Verification items for the finished model (mm, model axes). A direction names the side the tool comes from. Coordinates: 2 decimals unless noted, no trailing zeros. Order: outer loops, then holes, each group sorted by start corner. A loop starts at its lowest first (then second) coordinate and runs counter-clockwise, first axis right, second up. Notation, with made-up numbers: (66.5, 74) -> (80.5, 74) arc R22 ccw to (80.5, 85) -> close; hole circle Ø5 at (-21, -33). An arc over 180 degrees is marked (long way). Use CSV: the item, a comma, the result in double quotes. Start each with the question number.
1) Tool access check on faces 4 (the flat face through (-2, -36, 7)), 5 (the flat face through (-1, 3, -6)), 6 (the flat face through (49, -36, -8)), 7 (the cylindrical face through (44.536, 1.521, -6.325)). Record the directions out of +Z, -Z, +X, -X, +Y, -Y that give a thin tool (end or side, any length) a straight path to the whole face; none if there is none.
2) Scan lines: line 1 along X through (y, z) = (1.15, -6); line 2 along Y through (x, z) = (47.8, -5); line 3 along Y through (x, z) = (-37.5, -2.5). Record each from-to range of solid material in increasing order.
3) Sectioned sample at D-D on y = -37. Record the boundary of the cut face in (x, z), then the cut area to 3 significant figures.
4) Release check for a two-part mould opening along Y. For faces 1 (the cylindrical face through (-41.11, -60.03, 8.52)), 2 (the cylindrical face through (0.7, 2.39, 6.58)), 3 (the flat face through (-1, -38, 10)) record: released by +Y, released by -Y, zero draft, split by the parting line, or undercut.
5) Sectioned sample at C-C on z = 0.75. Record the boundary of the cut face in (x, y).
6) Sectioned sample at B-B on y = -55.27. Record the boundary of the cut face in (x, z), then the cut area to 3 significant figures.
7) Go/stop test with flat-tipped pins: pin 1 (2.5 mm diameter, centred on x = -23.5, y = -2, fed in from -Z); pin 2 (1.5 mm diameter, centred on x = 19, z = 5.5, fed in from -Y); pin 3 (1 mm diameter, centred on x = 38.5, z = -4, fed in from -Y); pin 4 (1.8 mm diameter, centred on x = -40, y = -61.04, fed in from +Z). Record where each tip stops, or that it passes through.
from build123d import *

# Parameters (mm, degrees)
SKETCH1_W           = 100
SKETCH1_H           = 20
BOSS_EXTRUDE1_DEPTH = 3
CUT_EXTRUDE1_REACH  = 53.078
SKETCH2_R           = 1.5
LPATTERN1_COUNT     = 2
LPATTERN1_PITCH     = 92
SKETCH3_W           = 100
SKETCH3_H           = 3
BOSS_EXTRUDE2_DEPTH = 68.54
SKETCH4_W           = 100
SKETCH4_H           = 5
BOSS_EXTRUDE3_DEPTH = 5
SKETCH5_W           = 100
SKETCH5_H           = 12
BOSS_EXTRUDE4_DEPTH = 3
FILLET4_R           = 12
SKETCH6_W           = 3
SKETCH6_H           = 63.54
BOSS_EXTRUDE5_DEPTH = 15
CUT_EXTRUDE2_REACH  = 123.646
SKETCH7_R           = 1.5
CUT_EXTRUDE3_REACH  = 89.165
SKETCH8_R           = 1.5
LPATTERN2_COUNT     = 2
LPATTERN2_PITCH     = 80


with BuildPart() as part:
    # Sketch1 → Boss-Extrude1 (new body)
    with BuildSketch(Plane(origin=(0, 0, 0), x_dir=(1, 0, 0), z_dir=(0, 1, 0))):
        Rectangle(SKETCH1_W, SKETCH1_H)
    extrude(amount=BOSS_EXTRUDE1_DEPTH)

    # Sketch2 → Cut-Extrude1 (cut, up to next)
    with BuildSketch(Plane(origin=(0, 3, 0), x_dir=(1, 0, 0), z_dir=(0, 1, 0)), mode=Mode.PRIVATE) as cut_extrude1_sk1:
        with Locations(Location((-46, 6, 0), (0, 0, 270))):
            Circle(SKETCH2_R)
    cut_extrude1_tool1 = extrude(cut_extrude1_sk1.sketch, amount=-CUT_EXTRUDE1_REACH, mode=Mode.PRIVATE) & part.part
    cut_extrude1 = cut_extrude1_tool1.solids().sort_by_distance((-46, 3, -6))[0]
    add(cut_extrude1, mode=Mode.SUBTRACT)

    # LPattern1: Cut-Extrude1 ×2
    with Locations(*[(i * LPATTERN1_PITCH, 0, 0) for i in range(1, LPATTERN1_COUNT)]):
        add(cut_extrude1, mode=Mode.SUBTRACT)

    # Sketch3 → Boss-Extrude2 (add)
    with BuildSketch(Plane.XZ):
        with Locations((0, 8.5)):
            Rectangle(SKETCH3_W, SKETCH3_H)
    extrude(amount=BOSS_EXTRUDE2_DEPTH)

    # Sketch4 → Boss-Extrude3 (add)
    with BuildSketch(Plane(origin=(0, 0, 7), x_dir=(-1, 0, 0), z_dir=(0, 0, -1))):
        with Locations((0, -2.5)):
            Rectangle(SKETCH4_W, SKETCH4_H)
    extrude(amount=BOSS_EXTRUDE3_DEPTH)

    # Sketch5 → Boss-Extrude4 (add)
    with BuildSketch(Plane(origin=(0, 3, 0), x_dir=(1, 0, 0), z_dir=(0, 1, 0))):
        with Locations((0, -4)):
            Rectangle(SKETCH5_W, SKETCH5_H)
    extrude(amount=BOSS_EXTRUDE4_DEPTH)

    # Fillet4
    fillet4_edges = [part.edges().sort_by_distance(p)[0] for p in [
        (0, 6, 10),
    ]]
    fillet(fillet4_edges, radius=FILLET4_R - 0.0001)  # a hair under: the kernel refuses the full size

    # Sketch6 → Boss-Extrude5 (add)
    with BuildSketch(Plane(origin=(0, 0, 7), x_dir=(-1, 0, 0), z_dir=(0, 0, -1))):
        with Locations((-48.5, -36.77)):
            Rectangle(SKETCH6_W, SKETCH6_H)
    extrude(amount=BOSS_EXTRUDE5_DEPTH)

    # Sketch7 → Cut-Extrude2 (cut, up to next)
    with BuildSketch(Plane(origin=(50, 0, 0), x_dir=(0, 0, -1), z_dir=(1, 0, 0)), mode=Mode.PRIVATE) as cut_extrude2_sk1:
        with Locations((5, -10.27)):
            Circle(SKETCH7_R)
    cut_extrude2_tool1 = extrude(cut_extrude2_sk1.sketch, amount=-CUT_EXTRUDE2_REACH, mode=Mode.PRIVATE) & part.part
    # Sketch7 → Cut-Extrude2 (cut, up to next)
    with BuildSketch(Plane(origin=(50, 0, 0), x_dir=(0, 0, -1), z_dir=(1, 0, 0)), mode=Mode.PRIVATE) as cut_extrude2_sk2:
        with Locations((5, -55.27)):
            Circle(SKETCH7_R)
    cut_extrude2_tool2 = extrude(cut_extrude2_sk2.sketch, amount=-CUT_EXTRUDE2_REACH, mode=Mode.PRIVATE) & part.part
    add(cut_extrude2_tool1.solids().sort_by_distance((50, -10.27, -5))[0], mode=Mode.SUBTRACT)
    add(cut_extrude2_tool2.solids().sort_by_distance((50, -55.27, -5))[0], mode=Mode.SUBTRACT)

    # Sketch8 → Cut-Extrude3 (cut, up to next)
    with BuildSketch(Plane.XY.offset(10), mode=Mode.PRIVATE) as cut_extrude3_sk1:
        with Locations((-40, -61.04)):
            Circle(SKETCH8_R)
    cut_extrude3_tool1 = extrude(cut_extrude3_sk1.sketch, amount=-CUT_EXTRUDE3_REACH, mode=Mode.PRIVATE) & part.part
    cut_extrude3 = cut_extrude3_tool1.solids().sort_by_distance((-40, -61.04, 10))[0]
    add(cut_extrude3, mode=Mode.SUBTRACT)

    # LPattern2: Cut-Extrude3 ×2
    with Locations(*[(i * LPATTERN2_PITCH, 0, 0) for i in range(1, LPATTERN2_COUNT)]):
        add(cut_extrude3, mode=Mode.SUBTRACT)


solid = part.part
Answers follow:
1,face 4,"-Z, -X, -Y"
1,face 5,"-Z, +X, -X, +Y"
1,face 6,"-Z, +X, -X, -Y"
1,face 7,"+Y"
2,line 1,"x = -50 to -47.5, -44.5 to 44.5, 47.5 to 50"
2,line 2,"y = -68.54 to -56.77, -53.77 to -11.77, -8.77 to -5, 0 to 3"
2,line 3,"y = 0 to 3"
3,outline,"(-50, 7) -> (47, 7) -> (47, -8) -> (50, -8) -> (50, 10) -> (-50, 10) -> close"
3,area,"345 mm²"
4,face 1,"undercut"
4,face 2,"released by +Y"
4,face 3,"zero draft"
5,outline,"(-50, 0) -> (50, 0) -> (50, 5.68) -> (-50, 5.68) -> close; (47, -68.54) -> (50, -68.54) -> (50, -5) -> (47, -5) -> close"
6,outline,"(-50, 7) -> (47, 7) -> (47, -3.5) -> (50, -3.5) -> (50, 10) -> (-50, 10) -> close; (47, -8) -> (50, -8) -> (50, -6.5) -> (47, -6.5) -> close"
6,area,"336 mm²"
7,pin 1,"stops at z = 2"
7,pin 2,"stops at y = -5"
7,pin 3,"stops at y = 0"
7,pin 4,"passes through"
